```python
from build123d import *

# Parameters (mm, degrees)
F1_DEPTH = 75
F2_R     = 2.95
F3_DEPTH = 5
F4_DEPTH = 3
F5_R     = 5
F6_SIZE  = 1.5


with BuildPart() as f1:
    # F0 (on Right) → F1 (new body)
    with BuildSketch(Plane.YZ):
        Polygon((0, 14.4), (0, 20.4), (-8, 20.4), (-8, -5), (0, -5), (0, -33.45), (8.4, -33.45), (8.4, -27.45), (4.4, -27.45), (4.4, 0), (0, 0), (0, 2.8), (-3, 2.8), (-3, 14.4), align=None)
    extrude(amount=F1_DEPTH)

    # F2 (on face) → F3 (cut, through all)
    with BuildSketch(Plane(origin=(0, -3, 0), x_dir=(-1, 0, 0), z_dir=(0, 1, 0))):
        with Locations((-59.7, 8.6)):
            Circle(F2_R)
        with Locations((-15.3, 8.6)):
            Circle(F2_R)
    extrude(amount=-F3_DEPTH, mode=Mode.SUBTRACT)

    # F2 (on face) → F4 (join, through all)
    with BuildSketch(Plane(origin=(0, -3, 0), x_dir=(-1, 0, 0), z_dir=(0, 1, 0))):
        with BuildLine():
            Line((-75, 2.8), (-59.7, 2.8))
            ThreePointArc((-59.7, 2.8), (-65.5, 8.6), (-59.7, 14.4))
            Line((-59.7, 14.4), (-75, 14.4))
            Line((-75, 14.4), (-75, 2.8))
        make_face()
        with BuildLine():
            Line((-15.3, 2.8), (0, 2.8))
            Line((0, 2.8), (0, 14.4))
            Line((0, 14.4), (-15.3, 14.4))
            ThreePointArc((-15.3, 14.4), (-11.198781, 12.701219), (-9.5, 8.6))
            ThreePointArc((-9.5, 8.6), (-11.198781, 4.498781), (-15.3, 2.8))
        make_face()
        with BuildLine():
            Line((-59.7, 2.8), (-15.3, 2.8))
            ThreePointArc((-15.3, 2.8), (-21.1, 8.6), (-15.3, 14.4))
            Line((-15.3, 14.4), (-59.7, 14.4))
            ThreePointArc((-59.7, 14.4), (-55.598781, 12.701219), (-53.9, 8.6))
            ThreePointArc((-53.9, 8.6), (-55.598781, 4.498781), (-59.7, 2.8))
        make_face()
    extrude(amount=F4_DEPTH)

    # F5
    f5_edges = [f1.edges().sort_by_distance(p)[0] for p in [
        (37.5, -8, 20.4),
        (37.5, -8, -5),
        (37.5, 0, -33.45),
    ]]
    fillet(f5_edges, radius=F5_R)

    # F6
    f6_edges = [f1.edges().sort_by_distance(p)[0] for p in [
        (18.25, -8, 8.6),
        (62.65, -8, 8.6),
    ]]
    chamfer(f6_edges, length=F6_SIZE)


solid = f1.part
```
Model file for the job. Use its own axes, mm. A direction names the side the tool comes from. Coordinates: 2 decimals unless noted, no trailing zeros. Order: outer loops, then holes, each group sorted by start corner. A loop starts at its lowest first (then second) coordinate and runs counter-clockwise, first axis right, second up. Notation, with made-up numbers: (8.5, 82) - (13.5, 82) arc R29 cw to (13.5, 109) - close; hole circle Ø11 at (77, 43). An arc over 180 degrees is marked (long way). Return JSON: item names as keys, results as strings. Group by question number.
1) Saw through at D-D, the plane z = -1. Write the cut outline in (x, y), plus the area to 3 significant figures.
2) Mould opens along X. For faces 1 (the flat face through (0, 2, -6)), 2 (the flat face through (57, -3, 7)), 3 (the flat face through (37, 7, -33.45)), 4 (the cylindrical face through (56.886, -4.726, 9.486)) say: released by +X, released by -X, zero draft, split by the parting line, or undercut.
3) Saw through at B-B, the plane x = 32.5. Write the cut outline in (y, z).
4) Saw through at A-A, the plane y = -1.5. Write the cut outline in (x, z), plus the area to 3 significant figures.
5) Flat gauge pins, fed straight in: P1, Ø22.5, axis at x = 20.5, z = 7.5, coming from the +Y side; P2, Ø4.5, axis at x = 42.5, y = 6.5, coming from the +Z side; P3, Ø4, axis at x = 61.5, z = -6, coming from the -Y side. Where does each tip first touch, or does it go through?
6) Saw through at C-C, the plane y = 6.75. Write the cut outline in (x, z), plus the area to 3 significant figures.
7) Probe line 1 (Z direction, x = 67.5, y = -0.75); line 2 (Z direction, x = 15.3, y = -4.9); line 3 (Y direction, x = 55, z = -22.5). List the from-to ranges inside material, lowest first. Write a range as from..to.
8) Tool access for faces 5 (the flat face through (38, 0, 10)), 6 (the flat face through (37, 8.4, -30)), 7 (the flat face through (18, -3, 11)), 8 (the flat face through (37, -2, -5)), 9 (the flat face through (37, -1, 20.4)): list every direction of +Z, -Z, +X, -X, +Y, -Y with a clear straight run to the whole face (end or side of a thin tool).
Values found:
{
 "1": {"outline": "(0, -7.9) - (75, -7.9) - (75, 4.4) - (0, 4.4) - close", "area": "922 mm²"},
 "2": {"face 1": "released by -X", "face 2": "undercut", "face 3": "zero draft", "face 4": "undercut"},
 "3": {"outline": "(-8, 0) arc R5 ccw to (-3, -5) - (0, -5) - (0, -28.45) arc R5 ccw to (5, -33.45) - (8.4, -33.45) - (8.4, -27.45) - (4.4, -27.45) - (4.4, 0) - (0, 0) - (0, 20.4) - (-3, 20.4) arc R5 ccw to (-8, 15.4) - close"},
 "4": {"outline": "(0, -5) - (75, -5) - (75, 20.4) - (0, 20.4) - close; hole (9.5, 8.6) arc R5.8 ccw to (15.3, 2.8) arc R5.8 ccw to (15.3, 14.4) arc R5.8 ccw to start; hole (53.9, 8.6) arc R5.8 ccw to (59.7, 2.8) arc R5.8 ccw to (59.7, 14.4) arc R5.8 ccw to start", "area": "1,690 mm²"},
 "5": {"P1": "stops at y = 4.4", "P2": "stops at z = 0", "P3": "stops at y = -6"},
 "6": {"outline": "(0, -33.45) - (75, -33.45) - (75, -27.45) - (0, -27.45) - close", "area": "450 mm²"},
 "7": {"line 1": "z = -5..20.4", "line 2": "z = -4.62..5.65, 11.55..20.02", "line 3": "y = 0..4.4"},
 "8": {"face 5": "+Z, +X, -X, +Y", "face 6": "+Z, -Z, +X, -X, +Y", "face 7": "+Y", "face 8": "-Z, +X, -X, -Y", "face 9": "+Z, +X, -X, +Y, -Y"}
}
